from build123d import *

# Parameters (mm, degrees)
SKETCH1_R           = 58.25
BOSS_EXTRUDE1_DEPTH = 6.9
SKETCH2_R           = 2
CUT_EXTRUDE1_DEPTH  = 6.9
SKETCH3_R           = 46.5
BOSS_EXTRUDE2_DEPTH = 30
SKETCH4_R           = 34
BOSS_EXTRUDE3_DEPTH = 33


with BuildPart() as part:
    # Sketch1 → Boss-Extrude1 (new body)
    with BuildSketch(Plane(origin=(0, 0, 0), x_dir=(1, 0, 0), z_dir=(0, 1, 0))):
        with Locations(Location((0, 0, 0), (0, 0, 90))):
            Circle(SKETCH1_R)
    extrude(amount=BOSS_EXTRUDE1_DEPTH)

    # Sketch2 → Cut-Extrude1 (cut)
    with BuildSketch(Plane(origin=(0, 6.9, 0), x_dir=(1, 0, 0), z_dir=(0, 1, 0))):
        with Locations(Location((0, 54, 0), (0, 0, 270))):
            Circle(SKETCH2_R)
        with Locations(Location((-54, 0, 0), (0, 0, 270))):
            Circle(SKETCH2_R)
        with Locations(Location((0, -54, 0), (0, 0, 270))):
            Circle(SKETCH2_R)
        with Locations(Location((54, 0, 0), (0, 0, 270))):
            Circle(SKETCH2_R)
    extrude(amount=-CUT_EXTRUDE1_DEPTH, mode=Mode.SUBTRACT)

    # Sketch3 → Boss-Extrude2 (add)
    with BuildSketch(Plane(origin=(0, 6.9, 0), x_dir=(1, 0, 0), z_dir=(0, 1, 0))):
        with Locations(Location((0, 0, 0), (0, 0, 270))):
            Circle(SKETCH3_R)
    extrude(amount=BOSS_EXTRUDE2_DEPTH)

    # Sketch4 → Boss-Extrude3 (add)
    with BuildSketch(Plane(origin=(0, 36.9, 0), x_dir=(1, 0, 0), z_dir=(0, 1, 0))):
        with Locations(Location((0, 0, 0), (0, 0, 270))):
            Circle(SKETCH4_R)
    extrude(amount=BOSS_EXTRUDE3_DEPTH)


solid = part.part
Read the model definition and answer for the solid it produces. Units are mm, in the model's axes. A direction names the side the tool comes from. Round coordinates to 2 decimals unless told otherwise and drop trailing zeros. Write each loop counter-clockwise with the first axis right and the second up, starting at its lowest first coordinate (ties: lowest second). Pieces come first, ordered by that corner, then holes.
1. Given pin 1 Ø10 at (x, y) = (43.5, 7.5) entering from +Z; pin 2 Ø2 at (y, z) = (24, -1) entering from -X; pin 3 Ø10 at (x, z) = (-43.5, -11) entering from +Y, each flat-ended and moving along its own axis, determine where each tip first touches the part or whether it passes through.
2. Determine the mould class of faces 3 (the face through (33.71, 53.17, -4.43)), 4 (the face through (-34.2, 36.9, 3.2)), 5 (the face through (0, 3, 52)) for opening direction Z: pulls with the +Z half, pulls with the -Z half, needs draft (parallel to the pull), parting line crosses it, or undercut.
3. The part is cut by section D-D, the plane y = 5. Determine the outline of the cut face in (x, z), then the cut area to 3 significant figures.
4. Straight lines are drawn through the part: L1, parallel to X at y = 2, z = 0; L2, parallel to Y at x = -11, z = 44; L3, parallel to Y at x = 49, z = -23.5. For each, find the intervals that lie inside material, in ascending order.
5. The part is cut by section B-B, the plane x = -54. Determine the outline of the cut face in (y, z), then the cut area to 3 significant figures.
6. Which of the six approach directions +Z, -Z, +X, -X, +Y, -Y give full straight-line access (tool end or side, diameter ignored) to faces 1 (the face through (46.1, 21.7, -6.1)), 2 (the face through (35.44, 3.4, 46.23))?
7. The part is cut by section C-C, the plane z = -54. Determine the outline of the cut face in (x, y).
8. The part is cut by section A-A, the plane z = 0. Determine the outline of the cut face in (x, y), then the cut area to 3 significant figures.
Values:
1. pin 1: stops at z = 43.68
1. pin 2: stops at x = -46.5
1. pin 3: stops at y = 36.9
2. face 3: parting line crosses it
2. face 4: needs draft
2. face 5: undercut
3. outline: circle Ø116.5 at (0, 0); hole circle Ø4 at (-54, 0); hole circle Ø4 at (0, -54); hole circle Ø4 at (0, 54); hole circle Ø4 at (54, 0)
3. area: 10,600 mm2
4. L1: x = -58.25 to -56, -52 to 52, 56 to 58.25
4. L2: y = 0 to 36.9
4. L3: y = 0 to 6.9
5. outline: (0, -21.84) - (6.9, -21.84) - (6.9, -2) - (0, -2) - close; (0, 2) - (6.9, 2) - (6.9, 21.84) - (0, 21.84) - close
5. area: 274 mm2
6. face 1: +Y
6. face 2: +Y, -Y
7. outline: (-21.84, 0) - (-2, 0) - (-2, 6.9) - (-21.84, 6.9) - close; (2, 0) - (21.84, 0) - (21.84, 6.9) - (2, 6.9) - close
8. outline: (-58.25, 0) - (-56, 0) - (-56, 6.9) - (-58.25, 6.9) - close; (-52, 0) - (52, 0) - (52, 6.9) - (46.5, 6.9) - (46.5, 36.9) - (34, 36.9) - (34, 69.9) - (-34, 69.9) - (-34, 36.9) - (-46.5, 36.9) - (-46.5, 6.9) - (-52, 6.9) - close; (56, 0) - (58.25, 0) - (58.25, 6.9) - (56, 6.9) - close
8. area: 5,780 mm2
